Solid Edge part; units mm, degrees
sketch "Sketch1" plane through (0, 0, 0) normal (1, 0, 0) x (0, 1, 0)
  circle A0 centre (0, 0) radius 10
extrude "Protrusion1" add sketch "Sketch1" along normal blind 7
sketch "Sketch2" plane through (7, 0, 0) normal (1, 0, 0) x (0, 1, 0)
  circle A0 centre (0, 5) radius 10
extrude "ExtrudedProtrusion_2" add sketch "Sketch2" along normal blind 4
sketch "Sketch3" plane through (11, 0, 5) normal (1, 0, 0) x (0, 1, 0)
  circle A0 centre (0, 0) radius 7
extrude "ExtrudedProtrusion_3" add sketch "Sketch3" along normal blind 19
sketch "Sketch4" plane through (30, 0, 5) normal (1, 0, 0) x (0, 1, 0)
  circle A0 centre (0, 0) radius 3
extrude "ExtrudedCutout_1" cut sketch "Sketch4" against normal blind 61.3249
chamfer "Chamfer_2" distance 0.5 angle 45 2 edges at (0, 3, 5) (30, -3, 5) measured on face at (5.3, 1.6602, 7.4988)
sketch "Sketch5" plane through (0, 0, 10.2) normal (0, 0, 1) x (1, 0, 0)
  line L0 (31, 2.5) -> (31, -2.5)
  line L1 (31, -2.5) -> (16, -2.5)
  arc A0 (16, -2.5) -> (16, 2.5) centre (16, 0) cw
  line L2 (16, 2.5) -> (31, 2.5)
extrude "ExtrudedCutout_2" cut sketch "Sketch5" along normal blind 26.2819
Source: CAD feature listing. Evaluate the final solid. Frame: model axes, mm. A direction names the side the tool comes from. Round coordinates to 2 decimals unless told otherwise and drop trailing zeros. Order: outer loops, then holes, each group sorted by start corner. A loop starts at its lowest first (then second) coordinate and runs counter-clockwise, first axis right, second up. Notation, with made-up numbers: (-6.75, 61.5) -> (8.25, 61.5) arc R35 ccw to (8.25, 95.5) -> close; hole circle Ø3 at (44.5, -37.5). An arc over 180 degrees is marked (long way). Use CSV: the item, a comma, the result in double quotes.
(1) Section C-C on x = 19. Return the cut outline in (y, z), and give its area (3 significant figures).
Report:
outline,"(-2.5, 10.2) -> (-2.5, 11.54) arc R7 ccw (long way) to (2.5, 11.54) -> (2.5, 10.2) -> close; hole circle Ø6 at (0, 5)"
area,"117 mm^2"
(2) Ray query, L1, parallel to Z at x = 7.25, y = 0; L2, parallel to Z at x = 15.25, y = 0; L3, parallel to Y at x = 4, z = 7. Return the intervals inside material, ascending.
Report:
L1,"-5 to 2, 8 to 15"
L2,"-2 to 2, 8 to 10.2"
L3,"-7.14 to -2.24, 2.24 to 7.14"
(3) Section D-D on z = 0. Return the cut outline in (x, y), and give its area (3 significant figures).
Report:
outline,"(0, -10) -> (7, -10) -> (7, -8.66) -> (11, -8.66) -> (11, -4.9) -> (30, -4.9) -> (30, 4.9) -> (11, 4.9) -> (11, 8.66) -> (7, 8.66) -> (7, 10) -> (0, 10) -> close"
area,"395 mm^2"
(4) Section B-B on z = 5. Return the cut outline in (x, y).
Report:
outline,"(0, -8.66) -> (7, -8.66) -> (7, -10) -> (11, -10) -> (11, -7) -> (30, -7) -> (30, -3.5) -> (29.5, -3) -> (0.5, -3) -> (0, -3.5) -> close; (0, 3.5) -> (0.5, 3) -> (29.5, 3) -> (30, 3.5) -> (30, 7) -> (11, 7) -> (11, 10) -> (7, 10) -> (7, 8.66) -> (0, 8.66) -> close"
(5) Access query for faces 1 (the face through (8.972, 4.614, 13.872)), 2 (the face through (7, 0, 11)), 3 (the face through (23, -2.5, 11)), 4 (the face through (7, -0.1, -5.2)). Directions: +Z, -Z, +X, -X, +Y, -Y. A direction counts if a zero-diameter tool reaches every point of the face in a straight line with its end or side. Return the directions, or none.
Report:
face 1,"+X"
face 2,"+Z, -X"
face 3,"+Z, +X"
face 4,"-Z, +X"
(6) Section A-A on y = 0. Return the cut outline in (x, z).
Report:
outline,"(0, -10) -> (7, -10) -> (7, -5) -> (11, -5) -> (11, -2) -> (30, -2) -> (30, 1.5) -> (29.5, 2) -> (0.5, 2) -> (0, 1.5) -> close; (0, 8.5) -> (0.5, 8) -> (29.5, 8) -> (30, 8.5) -> (30, 10.2) -> (13.5, 10.2) -> (13.5, 12) -> (11, 12) -> (11, 15) -> (7, 15) -> (7, 10) -> (0, 10) -> close"
(7) First-contact query: pin 1 Ø1.5 at (x, z) = (23.5, 11) entering from -Y; pin 2 Ø1 at (y, z) = (2, 4.5) entering from +X; pin 3 Ø5.5 at (x, y) = (20, 1) entering from +Z; pin 4 Ø1 at (x, z) = (20.5, -1) entering from -Y. Flat tips, straight axial feed; report the tip coordinate or a pass-through.
Report:
pin 1,"y = -4.63"
pin 2,"through"
pin 3,"z = 11.54"
pin 4,"y = -4.33"
